Print and shaded views of the part. All mm, measured from the part's lowest x, y and z. A direction names the side the tool comes from. Give positions to 0.01 mm unless a question says otherwise; leave off trailing zeros. Loops run counter-clockwise (first coordinate to the right, second up) from the corner with the lowest first, then second, coordinate; pieces in that order, holes last.
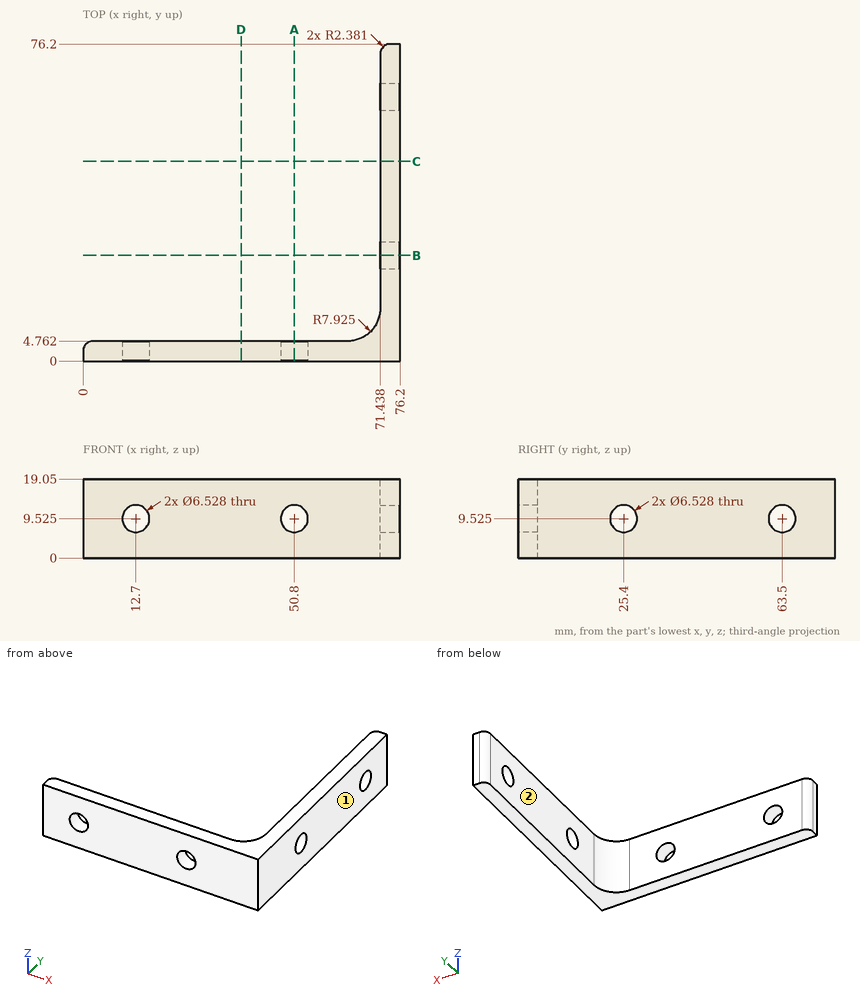
1. Saw through at C-C, the plane y = 48. List the corners of the cut face in (x, z).
Responses:
outline: (71.44, 0) - (76.2, 0) - (76.2, 19.05) - (71.44, 19.05) - close
2. Saw through at B-B, the plane y = 25.4. List the corners of the cut face in (x, z).
Responses:
outline: (71.44, 0) - (76.2, 0) - (76.2, 6.26) - (71.44, 6.26) - close; (71.44, 12.79) - (76.2, 12.79) - (76.2, 19.05) - (71.44, 19.05) - close
3. Tool access for the marked faces 1 and 2: list every direction of +Z, -Z, +X, -X, +Y, -Y with a clear straight run to the whole face (end or side of a thin tool).
Responses:
face 1: +Z, -Z, +X, +Y, -Y
face 2: +Z, -Z, -X, +Y
4. Drop flat-ended pins along their axis: pin 1 (4 mm diameter, centred on x = 52.5, z = 12, fed in from +Y); pin 2 (5.5 mm diameter, centred on y = 45.5, z = 12, fed in from -X). Give the stop position or say it passes through.
Responses:
pin 1: stops at y = 4.76
pin 2: stops at x = 71.44
5. Probe line 1 along Z through (x, y) = (74.35, 25.4); line 2 along Y through (x, z) = (39, 12.5); line 3 along X through (y, z) = (69.5, 8). List the from-to ranges inside material, lowest first.
Responses:
line 1: z = 0 to 6.26, 12.79 to 19.05
line 2: y = 0 to 4.76
line 3: x = 71.44 to 76.2
6. Saw through at D-D, the plane x = 38. List the corners of the cut face in (y, z).
Responses:
outline: (0, 0) - (4.76, 0) - (4.76, 19.05) - (0, 19.05) - close
7. Saw through at A-A, the plane x = 50.8. List the corners of the cut face in (y, z).
Responses:
outline: (0, 0) - (4.76, 0) - (4.76, 6.26) - (0, 6.26) - close; (0, 12.79) - (4.76, 12.79) - (4.76, 19.05) - (0, 19.05) - close
